```python
from build123d import *

# Parameters (mm, degrees)
SKETCH1_R           = 15
BOSS_EXTRUDE1_DEPTH = 44
SKETCH4_R           = 10
BOSS_EXTRUDE2_DEPTH = 5.5
BOSS_EXTRUDE3_START = 5.5
SKETCH5_R           = 10
BOSS_EXTRUDE3_DEPTH = 5.5


with BuildPart() as part:
    # Sketch1 → Boss-Extrude1 (new body)
    with BuildSketch(Plane.XY):
        Circle(SKETCH1_R)
    extrude(amount=BOSS_EXTRUDE1_DEPTH)

    # Sketch4 → Boss-Extrude2 (add)
    with BuildSketch(Plane.XY.offset(44)):
        Circle(SKETCH4_R)
    extrude(amount=BOSS_EXTRUDE2_DEPTH)

    # Sketch5 → Boss-Extrude3 (add)
    with BuildSketch(Plane(origin=(0, 0, 0), x_dir=(-1, 0, 0), z_dir=(0, 0, -1)).offset(BOSS_EXTRUDE3_START)):
        with Locations(Location((0, 0, 0), (0, 0, 180))):
            Circle(SKETCH5_R)
    extrude(amount=-BOSS_EXTRUDE3_DEPTH)


solid = part.part
```
Check sheet for the modelled part. Datum: model origin and axes. Units: mm. A direction names the side the tool comes from. Give positions to 0.01 mm unless a question says otherwise; leave off trailing zeros. Order: outer loops, then holes, each group sorted by start corner. A loop starts at its lowest first (then second) coordinate and runs counter-clockwise, first axis right, second up. Notation, with made-up numbers: M 40.25,38.25 L 76.25,38.25 A15 ccw 76.25,61.25 Z; hole C 15,-40 d3. An arc over 180 degrees is marked long. Answer in a Markdown table with one row per item. Add a question column.
Q1. Sectioned sample at C-C, the plane z = 13. Record the boundary of the cut face in (x, y).
Q2. Sectioned sample at D-D, the plane y = -12. Record the boundary of the cut face in (x, z).
Q3. Access from +Z, -Z, +X, -X, +Y, -Y to the whole of each face (thin tool, end or side, straight path). Record for faces 1 (the flat face through (0, 0, -5.5)), 2 (the cylindrical face through (-10, 0, -3)).
Q4. Release check for a two-part mould opening along Z. For faces 3 (the flat face through (3, -10, 44)), 4 (the cylindrical face through (-2.17, -9.76, 46.71)), 5 (the flat face through (3, -10, 0)) record: released by +Z, released by -Z, zero draft, split by the parting line, or undercut.
Q5. Gauge pin test, flat ends, axial feed: pin 1 Ø8 at (x, z) = (9.5, 4.5) entering from -Y; pin 2 Ø5 at (x, z) = (-3, 22) entering from -Y; pin 3 Ø12 at (x, z) = (-8, 3.5) entering from +Y. Record the tip position at first contact, or that the pin passes through.
Q6. Thickness scan on L1, parallel to Z at x = 12.5, y = -7.75; L2, parallel to Y at x = -0.5, z = 33.5; L3, parallel to Y at x = -13.5, z = 43. Record the ranges inside material, lowest first.
Q7. Sectioned sample at A-A, the plane y = 0. Record the boundary of the cut face in (x, z), and give its area (3 significant figures).
Verdict:
| question | item | result |
|---|---|---|
| 1 | outline | C 0,0 d30 |
| 2 | outline | M -9,0 L 9,0 L 9,44 L -9,44 Z |
| 3 | face 1 | -Z, +X, -X, +Y, -Y |
| 3 | face 2 | -Z |
| 4 | face 3 | released by +Z |
| 4 | face 4 | zero draft |
| 4 | face 5 | released by -Z |
| 5 | pin 1 | y = -13.96 |
| 5 | pin 2 | y = -14.99 |
| 5 | pin 3 | y = 14.87 |
| 6 | L1 | 0 to 44 |
| 6 | L2 | -14.99 to 14.99 |
| 6 | L3 | -6.54 to 6.54 |
| 7 | outline | M -15,0 L -10,0 L -10,-5.5 L 10,-5.5 L 10,0 L 15,0 L 15,44 L 10,44 L 10,49.5 L -10,49.5 L -10,44 L -15,44 Z |
| 7 | area | 1,540 mm² |
